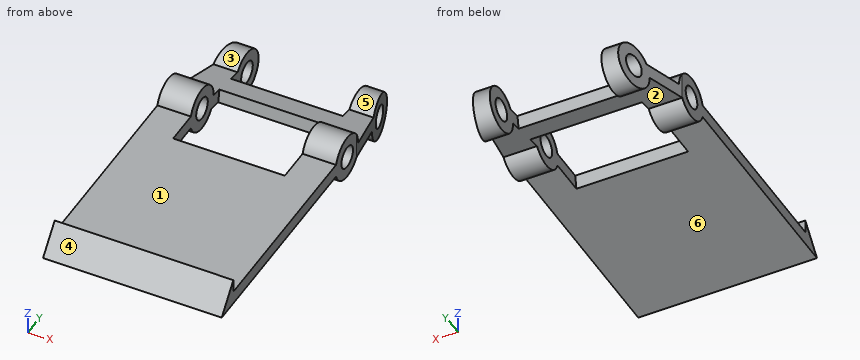
```python
from build123d import *

# Parameters (mm, degrees)
SKETCH1_R               = 2.5
BOSS_EXTRUDE1_DEPTH     = 20
CUT_EXTRUDE1_DEPTH      = 58.772252315
CUT_EXTRUDE1_DEPTH_BACK = 58.772252315
SKETCH2_W               = 25
SKETCH2_H               = 20
CUT_EXTRUDE2_DEPTH      = 58.772252315
CUT_EXTRUDE2_DEPTH_BACK = 58.772252315
SKETCH3_W               = 25
SKETCH3_H               = 12.433791975
CUT_EXTRUDE4_DEPTH      = 59.240774016
CUT_EXTRUDE4_DEPTH_BACK = 59.240774016


with BuildPart() as part:
    # Sketch1 → Boss-Extrude1 (new, symmetric)
    with BuildSketch(Plane(origin=(0, 0, 0), x_dir=(0, 1, 0), z_dir=(-1, 0, 0))):
        with BuildLine():
            Line((-54.034597787, 1.5), (-49, -4.5))
            Line((-49, -4.5), (-49, -1.5))
            Line((-49, -1.5), (-4.769696007, -1.5))
            ThreePointArc((-4.769696007, -1.5), (0.852265487, -4.926828954), (4.996412, 0.18938619))
            Line((4.996412, 0.18938619), (15.376256638, 1.98493936))
            ThreePointArc((15.376256638, 1.98493936), (24.074374147, 6.679586511), (14.368504731, 4.81061381))
            Line((14.368504731, 4.81061381), (3.988660093, 3.01506064))
            ThreePointArc((3.988660093, 3.01506064), (-0.852265487, 4.926828954), (-4.769696007, 1.5))
            Line((-4.769696007, 1.5), (-54.034597787, 1.5))
        make_face()
        with Locations(Location((0, 0, 0), (0, 0, 270))):
            Circle(SKETCH1_R, mode=Mode.SUBTRACT)
        with Locations(Location((19.364916731, 5, 0), (0, 0, 270))):
            Circle(SKETCH1_R, mode=Mode.SUBTRACT)
    extrude(amount=BOSS_EXTRUDE1_DEPTH, both=True)

    # Sketch2 → Cut-Extrude1 (cut, two sides: drawn at the far end of the back side and taken through both)
    with BuildSketch(Plane(origin=(0, -0.390517957, -2.25753032), x_dir=(-1, 0, 0), z_dir=(0, -0.17045309739797798, -0.9853657907535838)).offset(-CUT_EXTRUDE1_DEPTH_BACK)):
        with Locations((0, -2.5)):
            Rectangle(SKETCH2_W, SKETCH2_H)
    extrude(amount=CUT_EXTRUDE1_DEPTH + CUT_EXTRUDE1_DEPTH_BACK, mode=Mode.SUBTRACT)

    # Sketch3 → Cut-Extrude2 (cut, two sides: drawn at the far end of the back side and taken through both)
    with BuildSketch(Plane(origin=(0, -0.390517957, -2.25753032), x_dir=(-1, 0, 0), z_dir=(0, -0.17045309739797798, -0.9853657907535838)).offset(-CUT_EXTRUDE2_DEPTH_BACK)):
        with Locations((0, 18.716895988)):
            Rectangle(SKETCH3_W, SKETCH3_H)
    extrude(amount=CUT_EXTRUDE2_DEPTH + CUT_EXTRUDE2_DEPTH_BACK, mode=Mode.SUBTRACT)

    # Sketch4 → Cut-Extrude4 (cut, two sides: drawn at the far end of the back side and taken through both)
    with BuildSketch(Plane(origin=(0, 0, -1.5), x_dir=(-1, 0, 0), z_dir=(0, 0, -1)).offset(-CUT_EXTRUDE4_DEPTH_BACK)):
        Polygon((-20, 3.988660093), (-16.25, 24.364916731), (-20, 24.364916731), align=None)
        Polygon((20, 3.988660093), (20, 24.364916731), (16.25, 24.364916731), align=None)
    extrude(amount=CUT_EXTRUDE4_DEPTH + CUT_EXTRUDE4_DEPTH_BACK, mode=Mode.SUBTRACT)


solid = part.part
```
Geometry check sheet. Reference: the model listing, model coordinates, mm. Face numbers are marked on the shaded views. A direction names the side the tool comes from. Coordinates: 2 decimals unless noted, no trailing zeros. Order: outer loops, then holes, each group sorted by start corner. A loop starts at its lowest first (then second) coordinate and runs counter-clockwise, first axis right, second up.
Item 1: Section check C-C (z = -6). Enter the section's corners in (x, y).
Item 2: Mould release check, pull along Y, two halves, no side actions. Record for the marked faces 4, 5 and 6: released by +Y, released by -Y, zero draft, split by the parting line, or undercut.
Item 3: Section check D-D (y = -30). Enter the section's corners in (x, z), plus the area to 3 significant figures.
Item 4: Section check B-B (y = 0). Enter the section's corners in (x, z).
Item 5: Section check A-A (x = 0.5). Enter the section's corners in (y, z), plus the area to 3 significant figures.
Item 6: Depth check by flat-ended pin: pin 1 (4.5 mm diameter, centred on y = 0, z = 0, fed in from +X); pin 2 (8 mm diameter, centred on y = 16.5, z = -7, fed in from -X); pin 3 (8 mm diameter, centred on y = 19.36, z = -5, fed in from -X); pin 4 (5 mm diameter, centred on y = 20.5, z = -7, fed in from +X). Enter the tip coordinate at first touch or a pass-through.
Item 7: Tool access check on the marked faces 1, 2 and 3. Record the directions out of +Z, -Z, +X, -X, +Y, -Y that give a thin tool (end or side, any length) a straight path to the whole face; none if there is none.
Item 8: Scan lines: line 1 along Z through (x, y) = (14.5, 0); line 2 along Z through (x, y) = (-18, -11); line 3 along Y through (x, z) = (-5, 0). Record each from-to range of solid material in increasing order.
Check sheet entries:
1. outline: (-18.07, 14.47) - (-12.5, 14.47) - (-12.5, 17.07) - (-17.59, 17.07) - close; (-16.75, 21.66) - (-12.5, 21.66) - (-12.5, 24.26) - (-16.27, 24.26) - close; (12.5, 14.47) - (18.07, 14.47) - (17.59, 17.07) - (12.5, 17.07) - close; (12.5, 21.66) - (16.75, 21.66) - (16.27, 24.26) - (12.5, 24.26) - close
2. face 4: released by -Y
2. face 5: undercut
2. face 6: zero draft
3. outline: (-20, -1.5) - (20, -1.5) - (20, 1.5) - (-20, 1.5) - close
3. area: 120 mm2
4. outline: (-20, -5) - (-12.5, -5) - (-12.5, -2.5) - (-20, -2.5) - close; (-20, 2.5) - (-12.5, 2.5) - (-12.5, 5) - (-20, 5) - close; (12.5, -5) - (20, -5) - (20, -2.5) - (12.5, -2.5) - close; (12.5, 2.5) - (20, 2.5) - (20, 5) - (12.5, 5) - close
5. outline: (-54.03, -1.5) - (-12.95, -1.5) - (-12.43, 1.5) - (-49, 1.5) - (-49, 4.5) - close; (7, -3.54) - (11.93, -4.39) - (12.43, -1.48) - (7.5, -0.62) - close
5. area: 139 mm2
6. pin 1: passes through
6. pin 2: stops at x = -18.29
6. pin 3: stops at x = -17.91
6. pin 4: stops at x = 17.42
7. face 1: +Z, +X, -X
7. face 2: -Z, +X, -X
7. face 3: +X, -X
8. line 1: z = -5 to -2.5, 2.5 to 5
8. line 2: z = -1.5 to 1.5
8. line 3: y = -52.78 to -12.69
